Here's how the part is built. I have some questions about the finished solid (model axes, mm). Face numbers are marked on the shaded views. A direction names the side the tool comes from. Round coordinates to 2 decimals unless told otherwise and drop trailing zeros. Write each loop counter-clockwise with the first axis right and the second up, starting at its lowest first coordinate (ties: lowest second). Pieces come first, ordered by that corner, then holes. Notation, with made-up numbers: M 8,9.5 L 55,9.5 A13 ccw 55,19.5 Z; hole C 10,15.5 d9. An arc over 180 degrees is marked long. Write item = value, one per line. Start each with the question number.
(1) I want a section at B-B (y = 28.5). List the corners of the cut face in (x, z) for me.
(2) I need wall thicknesses on line 1 along Y through (x, z) = (4.5, -25); line 2 along Y through (x, z) = (2.5, -24); line 3 along Y through (x, z) = (-1, -23). Which ranges of each line are inside material? Lowest first, please.
(3) I want a section at C-C (x = 0.25). List the corners of the cut face in (y, z) for me.
(4) Will these pins go through, and if not, where does the flat tip stop? pin 1 Ø4 at (x, z) = (-0.5, -26) entering from -Y; pin 2 Ø6 at (x, y) = (-4.5, 5.5) entering from +Z; pin 3 Ø1.7 at (x, z) = (-3, -29.5) entering from +Y; pin 4 Ø3 at (x, y) = (1, 28.5) entering from -Z.
(5) On a 3-axis mill with a long thin cutter (end or side, diameter ignored), from which of +Z, -Z, +X, -X, +Y, -Y can I reach the whole of each face in a straight line? I mean the marked faces 4, 5, 6 and 7. Say none if no direction works.
(6) I want a section at A-A (z = -25). List the corners of the cut face in (x, y) for me, and give its area (3 significant figures).
(7) If we mould it in two halves opening along Y, with no side actions, what happens to the marked faces 1, 2 and 3? For each: released by +Y, released by -Y, zero draft, split by the parting line, or undercut.
(8) I want a section at D-D (x = 9). List the corners of the cut face in (y, z) for me.
```python
from build123d import *

# Parameters (mm, degrees)
BOSS_EXTRUDE1_DEPTH = 35
SKETCH2_W           = 22
SKETCH2_H           = 4.75
BOSS_EXTRUDE2_DEPTH = 6
SKETCH3_W           = 2.5
SKETCH3_H           = 2.5
BOSS_EXTRUDE3_DEPTH = 22
SKETCH4_W           = 22
SKETCH4_H           = 7.25
CUT_EXTRUDE1_DEPTH  = 1.8
SKETCH5_W           = 12
SKETCH5_H           = 5.357838174
CUT_EXTRUDE2_DEPTH  = 9.8


with BuildPart() as part:
    # Sketch1 → Boss-Extrude1 (new body)
    with BuildSketch(Plane(origin=(0, 0, 0), x_dir=(1, 0, 0), z_dir=(0, 1, 0))):
        with BuildLine():
            Line((-11, 27.910571474), (11, 27.910571474))
            ThreePointArc((11, 27.910571474), (0, 30), (-11, 27.910571474))
        make_face()
    extrude(amount=BOSS_EXTRUDE1_DEPTH)

    # Sketch2 → Boss-Extrude2 (add)
    with BuildSketch(Plane.XY.offset(-27.910571474)):
        with Locations((0, 32.625)):
            Rectangle(SKETCH2_W, SKETCH2_H)
        with Locations((0, 2.375)):
            Rectangle(SKETCH2_W, SKETCH2_H)
    extrude(amount=BOSS_EXTRUDE2_DEPTH)

    # Sketch3 → Boss-Extrude3 (add, through all)
    with BuildSketch(Plane.ZY.offset(11)):
        with Locations((-23.160571474, 29)):
            Rectangle(SKETCH3_W, SKETCH3_H)
        with Locations((-23.160571474, 6)):
            Rectangle(SKETCH3_W, SKETCH3_H)
    extrude(amount=-BOSS_EXTRUDE3_DEPTH)

    # Sketch4 → Cut-Extrude1 (cut)
    with BuildSketch(Plane.XY.offset(-21.910571474)):
        with Locations((0, 3.625)):
            Rectangle(SKETCH4_W, SKETCH4_H)
    extrude(amount=-CUT_EXTRUDE1_DEPTH, mode=Mode.SUBTRACT)

    # Sketch5 → Cut-Extrude2 (cut)
    with BuildSketch(Plane(origin=(0, 35, 0), x_dir=(1, 0, 0), z_dir=(0, 1, 0))):
        with Locations((0, 29.043466622)):
            Rectangle(SKETCH5_W, SKETCH5_H)
    extrude(amount=-CUT_EXTRUDE2_DEPTH, mode=Mode.SUBTRACT)


solid = part.part
```
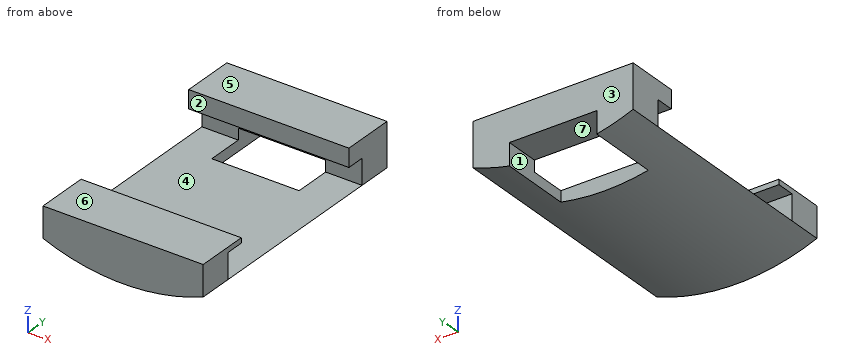
Returned:
q1.outline = M -11,-27.91 A30 ccw -6,-29.39 L -6,-27.91 Z; M -11,-24.41 L 11,-24.41 L 11,-21.91 L -11,-21.91 Z; M 6,-29.39 A30 ccw 11,-27.91 L 6,-27.91 Z
q2.line_1 = 0 to 4.75, 30.25 to 35
q2.line_2 = 0 to 7.25, 27.75 to 35
q2.line_3 = 27.75 to 35
q3.outline = M 0,-30 L 25.2,-30 L 25.2,-27.91 L 4.75,-27.91 L 4.75,-24.41 L 7.25,-24.41 L 7.25,-23.71 L 0,-23.71 Z; M 27.75,-24.41 L 30.25,-24.41 L 30.25,-26.36 L 35,-26.36 L 35,-21.91 L 27.75,-21.91 Z
q4.pin_1 = 0
q4.pin_2 = -23.71
q4.pin_3 = 25.2
q4.pin_4 = -24.41
q5.face_4 = +X, -X
q5.face_5 = +Z, +X, -X, +Y, -Y
q5.face_6 = +Z, +X, -X, -Y
q5.face_7 = -Z, +Y
q6.outline = M -11,0 L 11,0 L 11,4.75 L -11,4.75 Z; M -11,30.25 L 11,30.25 L 11,35 L -11,35 Z
q6.area = 209 mm²
q7.face_1 = zero draft
q7.face_2 = undercut
q7.face_3 = released by +Y
q8.outline = M 0,-28.62 L 35,-28.62 L 35,-21.91 L 27.75,-21.91 L 27.75,-24.41 L 30.25,-24.41 L 30.25,-27.91 L 4.75,-27.91 L 4.75,-24.41 L 7.25,-24.41 L 7.25,-23.71 L 0,-23.71 Z
